from build123d import *

# Parameters (mm, degrees)
SKETCH1_W                = 50
SKETCH1_H                = 50
BOSS_EXTRUDE1_DEPTH      = 50
CUT_SWEEP3_START         = 47
CUT_SWEEP3_DEPTH         = 3
CUT_SWEEP3_2_ANGLE       = 52.934263
SKETCH12_W               = 22
SKETCH12_H               = 36
CUT_EXTRUDE6_DEPTH       = 11
SKETCH13_W               = 22
SKETCH13_H               = 20.943650814
CUT_EXTRUDE7_DEPTH       = 20
SKETCH14_W               = 22
SKETCH14_H               = 7.504472325
CUT_EXTRUDE8_DEPTH       = 12
CHAMFER1_SIZE            = 1.5
BOSS_EXTRUDE2_DEPTH      = 7
BOSS_EXTRUDE2_DEPTH_BACK = 10
SKETCH15_W               = 1
SKETCH15_H               = 7
SKETCH16_W               = 1.8
SKETCH16_H               = 1.8
CUT_EXTRUDE9_DEPTH       = 7


with BuildPart() as part:
    # Sketch1 → Boss-Extrude1 (new body)
    with BuildSketch(Plane.XY):
        with Locations((25, 25)):
            Rectangle(SKETCH1_W, SKETCH1_H)
    extrude(amount=BOSS_EXTRUDE1_DEPTH)

    # Cut-Sweep3: read off the stored shape, not the designer's step
    # Cut-Sweep3 outline → Cut-Sweep3 (cut)
    with BuildSketch(Plane(origin=(0, 0, 0), x_dir=(1, 0, 0), z_dir=(0, 1, 0)).offset(CUT_SWEEP3_START)):
        Polygon((20.443650814, -39), (14, -45.443650814), (14, -50), (36, -50), (36, -45.443650814), (29.556349186, -39), align=None)
    extrude(amount=CUT_SWEEP3_DEPTH, mode=Mode.SUBTRACT)

    # Cut-Sweep3 2 outline → Cut-Sweep3 2 (revolve, cut)
    with BuildSketch(Plane(origin=(0, 47, 39), x_dir=(0, 0, 1), z_dir=(0, 1, 0))):
        Polygon((6.443650814, 14), (15.556349186, 14), (18.250266522, 16.693917336), (18.250266522, 33.306082664), (15.556349091, 36.000000095), (6.443650814, 36), (0, 29.556349186), (0, 20.443650814), align=None)
    revolve(axis=Axis((0, 47, 39), (1, 0, 0)), revolution_arc=CUT_SWEEP3_2_ANGLE, mode=Mode.SUBTRACT)

    # Cut-Sweep4: sweep along a path in Sketch9
    with BuildLine(Plane(origin=(25, 0, 0), x_dir=(0, 0, -1), z_dir=(1, 0, 0))) as cut_sweep4_path:
        Line((-13.5, 0), (-13.5, 3))
        ThreePointArc((-13.5, 3), (-15.805815997, 12.805055658), (-22.239919677, 20.554779117))
        Line((-22.239919677, 20.554779117), (-45.630040161, 38.222610442))
    # Sketch5<2> → Cut-Sweep4 (sweep, cut)
    with BuildSketch(Plane(origin=(25, 38.222610442, 45.630040161), x_dir=(-1, 0, 0), z_dir=(0, -0.6027309237648077, -0.7979445052994735))):
        Polygon((4.556349186, 11), (-4.556349186, 11), (-11, 4.556349186), (-11, -4.556349186), (-4.556349186, -11), (4.556349186, -11), (11, -4.556349186), (11, 4.556349186), align=None)
    sweep(path=cut_sweep4_path.line, mode=Mode.SUBTRACT)

    # Sketch12 → Cut-Extrude6 (cut)
    with BuildSketch(Plane.XY.offset(50)):
        with Locations((25, 18)):
            Rectangle(SKETCH12_W, SKETCH12_H)
    extrude(amount=-CUT_EXTRUDE6_DEPTH, mode=Mode.SUBTRACT)

    # Sketch13 → Cut-Extrude7 (cut)
    with BuildSketch(Plane.XZ):
        with Locations((25, 28.528174593)):
            Rectangle(SKETCH13_W, SKETCH13_H)
    extrude(amount=-CUT_EXTRUDE7_DEPTH, mode=Mode.SUBTRACT)

    # Sketch14 → Cut-Extrude8 (cut)
    with BuildSketch(Plane.XY.offset(39)):
        with Locations((25, 23.752236163)):
            Rectangle(SKETCH14_W, SKETCH14_H)
    extrude(amount=-CUT_EXTRUDE8_DEPTH, mode=Mode.SUBTRACT)

    # Chamfer1
    chamfer1_edges = [part.edges().sort_by_distance(p)[0] for p in [
        (50, 25, 50),
        (43, 0, 50),
        (43, 50, 50),
        (7, 50, 50),
        (14, 25, 50),
        (36, 18, 50),
        (14, 50, 47.721825407),
        (36, 50, 47.721825407),
        (32.778174593, 50, 42.221825407),
        (17.221825407, 50, 42.221825407),
        (0, 25, 50),
        (25, 50, 0),
        (50, 25, 0),
        (25, 0, 0),
        (0, 25, 0),
        (17.221825407, 0, 5.721825407),
        (32.778174593, 0, 5.721825407),
        (36, 0, 29.471825407),
        (14, 0, 29.471825407),
        (7, 0, 50),
        (0, 50, 25),
        (50, 50, 25),
        (50, 0, 25),
        (0, 0, 25),
    ]]
    chamfer(chamfer1_edges, length=CHAMFER1_SIZE)

    # Sketch15 → Boss-Extrude2 (add, two sides: drawn at the far end of the back side and taken through both)
    with BuildSketch(Plane.XY.offset(50).offset(-BOSS_EXTRUDE2_DEPTH_BACK)):
        with Locations((0.5, 25)):
            Rectangle(SKETCH15_W, SKETCH15_H)
    extrude(amount=BOSS_EXTRUDE2_DEPTH + BOSS_EXTRUDE2_DEPTH_BACK)

    # Sketch16 → Cut-Extrude9 (cut)
    with BuildSketch(Plane(origin=(1, 0, 0), x_dir=(0, 0, -1), z_dir=(1, 0, 0))):
        with Locations((-53.6, 25)):
            Rectangle(SKETCH16_W, SKETCH16_H)
    extrude(amount=-CUT_EXTRUDE9_DEPTH, mode=Mode.SUBTRACT)


solid = part.part
Model file for the job. Use its own axes, mm. A direction names the side the tool comes from. Give positions to 0.01 mm unless a question says otherwise; leave off trailing zeros. Write each loop counter-clockwise with the first axis right and the second up, starting at its lowest first coordinate (ties: lowest second). Pieces come first, ordered by that corner, then holes. Notation, with made-up numbers: (68.5, 21) -> (103.5, 21) arc R22 ccw to (103.5, 39) -> close; hole circle Ø1 at (-18.5, 4). An arc over 180 degrees is marked (long way). Write item = value, one per line.
(1) Slice it at C-C, the plane z = 29.5. Give the cut face in (x, y).
Determined:
outline = (0, 1.5) -> (1.5, 0) -> (12.5, 0) -> (14, 1.5) -> (14, 31.75) -> (20.44, 39.82) -> (29.56, 39.82) -> (36, 31.75) -> (36, 1.5) -> (37.5, 0) -> (48.5, 0) -> (50, 1.5) -> (50, 48.5) -> (48.5, 50) -> (1.5, 50) -> (0, 48.5) -> close
(2) Flat gauge pins, fed straight in: P1, Ø1.1, axis at x = 0.5, z = 53.5, coming from the +Y side; P2, Ø2, axis at y = 23.5, z = 52, coming from the +X side; P3, Ø1.1, axis at x = 0.5, z = 53.5, coming from the -Y side. Where does each tip first touch, or does it go through?
Determined:
P1 = 28.5
P2 = 1
P3 = 21.5
(3) Tool access for faces 1 (the face through (36.7, 49.2, 46.7)), 2 (the face through (32.823, 47.74, 42.267)), 3 (the face through (32.733, 2.261, 5.677)): list every direction of +Z, -Z, +X, -X, +Y, -Y with a clear straight run to the whole face (end or side of a thin tool).
Determined:
face_1 = +Z, +Y
face_2 = +Z, +Y, -Y
face_3 = +Z, -Y
(4) Probe line 1 along X through (y, z) = (13.5, 34); line 2 along Z through (x, y) = (42.5, 28); line 3 along X through (y, z) = (29.5, 22). List the from-to ranges inside material, lowest first.
Determined:
line_1 = 0 to 14, 36 to 50
line_2 = 0 to 50
line_3 = 0 to 16.73, 33.27 to 50
(5) Mould opens along X. For faces 4 (the face through (24.7, 49.2, 0.7)), 5 (the face through (16.43, 0.76, 5.47)), 6 (the face through (0.8, 24.7, 0.7)) say: released by +X, released by -X, zero draft, split by the parting line, or undercut.
Determined:
face_4 = zero draft
face_5 = undercut
face_6 = released by -X
(6) Slice it at A-A, the plane z = 47. Give the cut face in (x, y).
Determined:
outline = (0, 1.5) -> (1.5, 0) -> (12.5, 0) -> (14, 1.5) -> (14, 48.5) -> (12.5, 50) -> (1.5, 50) -> (0, 48.5) -> close; (36, 1.5) -> (37.5, 0) -> (48.5, 0) -> (50, 1.5) -> (50, 48.5) -> (48.5, 50) -> (37.5, 50) -> (36, 48.5) -> close
(7) Slice it at B-B, the plane x = 46.5. Give the cut face in (y, z).
Determined:
outline = (0, 1.5) -> (1.5, 0) -> (48.5, 0) -> (50, 1.5) -> (50, 48.5) -> (48.5, 50) -> (1.5, 50) -> (0, 48.5) -> close
(8) Slice it at D-D, the plane x = 23.5. Give the cut face in (y, z).
Determined:
outline = (0, 1.5) -> (1.5, 0) -> (48.5, 0) -> (50, 1.5) -> (50, 39) -> (47, 39) -> (29.33, 15.61) arc R33 cw to (3, 2.5) -> (0, 2.5) -> close
